Autodesk Inventor part; units mm, degrees
ref_plane "Work Plane1" through (0, 0, -3.8225) normal (0, 0, 1) x (1, 0, 0)
ref_plane "YZ Plane" through (0, 0, 0) normal (1, 0, 0) x (0, 1, 0)
ref_plane "XZ Plane" through (0, 0, 0) normal (0, 1, 0) x (-1, 0, 0)
sketch "Sketch1" plane through (0, 0, 0) normal (1, 0, 0) x (0, 1, 0)
  line L0 (3.8225, -3.8225) -> (3.8225, -892.8225)
  arc A0 (3.8225, -3.8225) -> (0, 0) centre (0, -3.8225) ccw
  arc A1 (0, 0) -> (-3.8225, -3.8225) centre (0, -3.8225) ccw
  line L1 (-3.8225, -3.8225) -> (-3.8225, -892.8225)
  arc A2 (0, -896.645) -> (3.8225, -892.8225) centre (0, -892.8225) ccw
  arc A3 (-3.8225, -892.8225) -> (0, -896.645) centre (0, -892.8225) ccw
  line L2 (0, 0) -> (0, -7.645)
  line L3 (0, -889) -> (0, -896.645)
  dimension "d0" = 896.645
  dimension "d2" = 3.8225
  dimension "d3" = 3.8225
ref_plane "Work Plane1" through (0, 0, -3.8225) normal (0, 0, 1) x (1, 0, 0)
sketch "Sketch2" plane through (0, 0, -3.8225) normal (0, 0, 1) x (1, 0, 0)
  line L0 (-3, 5.8225) -> (3, 5.8225)
  line L1 (3, 5.8225) -> (3, 3.8225)
  line L2 (3, 3.8225) -> (-3, 3.8225)
  line L3 (-3, 3.8225) -> (-3, 5.8225)
  line L4 (0, 0) -> (0, 3.8225)
  point P0 (0, 0)
  point P1 (0, 5.8225)
  dimension "d5" = 2
  dimension "d6" = 0
  dimension "d7" = 6
sweep "Sweep1" add profiles "Sketch2" path "Sketch1" path curves L0 A2 A3 L1 A1 A0
properties part number "Carriage Belt"
Geometry check sheet. Reference: the model listing, model coordinates, mm. Give positions to 0.01 mm unless a question says otherwise; leave off trailing zeros. Order: outer loops, then holes, each group sorted by start corner. A loop starts at its lowest first (then second) coordinate and runs counter-clockwise, first axis right, second up. Notation, with made-up numbers: (19, 85.5) -> (28, 85.5) arc R8 ccw to (28, 94.5) -> close; hole circle Ø4 at (49, 27). An arc over 180 degrees is marked (long way). Write each question's results on one line, items separated by ' | '. Start each with the question number.
(1) Sectioned sample at B-B (y = 0). Enter the section's corners in (x, z) (3 decimals).
(2) Sectioned sample at A-A (z = -595). Enter the section's corners in (x, y).
(3) Sectioned sample at C-C (x = -1.7). Enter the section's corners in (y, z) (1 decimal), plus the area to 3 significant figures.
(4) Scan lines: line 1 (Y direction, x = 1.2, z = -131); line 2 (Z direction, x = -1.4, y = 4.5); line 3 (Z direction, x = 2.2, y = -1). Record each from-to range of solid material in increasing order.
Answer below:
1) outline: (-3, -898.645) -> (3, -898.645) -> (3, -896.645) -> (-3, -896.645) -> close; (-3, 0) -> (3, 0) -> (3, 2) -> (-3, 2) -> close
2) outline: (-3, -5.82) -> (3, -5.82) -> (3, -3.82) -> (-3, -3.82) -> close; (-3, 3.82) -> (3, 3.82) -> (3, 5.82) -> (-3, 5.82) -> close
3) outline: (-5.8, -892.8) arc R5.8 ccw to (5.8, -892.8) -> (5.8, -3.8) arc R5.8 ccw to (-5.8, -3.8) -> close; hole (-3.8, -892.8) arc R3.8 ccw to (3.8, -892.8) -> (3.8, -3.8) arc R3.8 ccw to (-3.8, -3.8) -> close | area: 3,620 mm2
4) line 1: -5.82 to -3.82, 3.82 to 5.82 | line 2: -896.52 to -0.13 | line 3: -898.56 to -896.51, -0.13 to 1.91
